For this review, take the finished solid that the model builds, in its own axes (mm). A direction names the side the tool comes from. Coordinates: 2 decimals unless noted, no trailing zeros. Write each loop counter-clockwise with the first axis right and the second up, starting at its lowest first coordinate (ties: lowest second). Pieces come first, ordered by that corner, then holes. Notation, with made-up numbers: (56.5, -31.75) -> (76.5, -31.75) arc R27 ccw to (76.5, -0.75) -> close; hole circle Ø1 at (74.5, -33.75). An arc over 180 degrees is marked (long way). Put each result on its own line as item: value. Start each with the question number.
Item 1: Insertion check: P1, Ø4, axis at x = 7.5, z = -8.5, coming from the +Y side; P2, Ø5, axis at x = 3.5, y = -11.5, coming from the -Z side; P3, Ø6, axis at x = 7, z = -3.5, coming from the -Y side. Each pin has a flat end and moves straight along its axis. Give the tip position at first contact, or say it passes through.
Item 2: For faces 4 (the flat face through (7, -8, -12)), 5 (the cylindrical face through (7.54, 0.07, -10.5)), 6 (the flat face through (0, 0, 8)), 7 (the flat face through (8, 8, -12)), 8 (the flat face through (5, -2, -12)), list the 3-axis set-ups (+Z, -Z, +X, -X, +Y, -Y) from which the entire face can be reached by the end or side of a thin tool; tool diameter is ignored.
Item 3: To check wall thickness, follow L1, parallel to Y at x = 0, z = 5.5; L2, parallel to X at y = -5, z = -18; L3, parallel to Z at x = 2.25, y = -11. State the ranges of each line that lie inside material, in increasing order.
Item 4: Consider section D-D on z = -6.5. Give the boundary of the cut face in (x, y), and give its area (3 significant figures).
Item 5: Consider section B-B on x = 0. Give the boundary of the cut face in (y, z), and give its area (3 significant figures).
Item 6: Consider section C-C on y = 0. Give the boundary of the cut face in (x, z).
Item 7: Consider section A-A on z = -12. Give the boundary of the cut face in (x, y), and give its area (3 significant figures).
Item 8: The part is to be moulded in two halves that separate along Y. For faces 1 (the flat face through (0, 30, 4)), 2 (the cylindrical face through (-7.46, 0.07, -10.5)), 3 (the flat face through (7, 0, -25)), say which applies: +Y half, -Y half, draft (parallel to the pull), parting line (faces both ways), or undercut.
```python
from build123d import *

# Parameters (mm, degrees)
SKETCH_1_W          = 20
SKETCH_1_H          = 60
SKETCH_1_R          = 3
EXTRUDE_1_DEPTH     = 8
EXTRUDE_3_DEPTH     = 25
SKETCH_4_R          = 1.5
CUT_EXTRUDE_1_DEPTH = 25


with BuildPart() as part:
    # 草图1 → 凸台-拉伸1 (new body)
    with BuildSketch(Plane.XY):
        Rectangle(SKETCH_1_W, SKETCH_1_H)
        with Locations((0, 15)):
            Circle(SKETCH_1_R, mode=Mode.SUBTRACT)
        with Locations((0, -15)):
            Circle(SKETCH_1_R, mode=Mode.SUBTRACT)
    extrude(amount=EXTRUDE_1_DEPTH)

    # 草图3 → 凸台-拉伸3 (add)
    with BuildSketch(Plane(origin=(0, 0, 0), x_dir=(-1, 0, 0), z_dir=(0, 0, -1))):
        Polygon((-5, -6), (-5, -8), (-10, -8), (-10, 8), (-5, 8), (-5, 6), align=None)
        Polygon((10, -8), (10, 8), (5, 8), (5, 6), (5, -6), (5, -8), align=None)
    extrude(amount=EXTRUDE_3_DEPTH)

    # 草图4 → 切除-拉伸1 (cut)
    with BuildSketch(Plane(origin=(10, 0, 0), x_dir=(0, 0, -1), z_dir=(1, 0, 0))):
        with Locations((12, 0)):
            Circle(SKETCH_4_R)
    extrude(amount=-CUT_EXTRUDE_1_DEPTH, mode=Mode.SUBTRACT)


solid = part.part
```
Return value:
1. P1: y = 8
1. P2: z = 0
1. P3: y = -8
2. face 4: -Z, +X, -X, -Y
2. face 5: +X, -X
2. face 6: +Z, +X, -X, +Y, -Y
2. face 7: -Z, +X, -X, +Y
2. face 8: -Z, +Y, -Y
3. L1: -30 to -18, -12 to 12, 18 to 30
3. L2: -10 to -5, 5 to 10
3. L3: 0 to 8
4. outline: (-10, -8) -> (-5, -8) -> (-5, 8) -> (-10, 8) -> close; (5, -8) -> (10, -8) -> (10, 8) -> (5, 8) -> close
4. area: 160 mm^2
5. outline: (-30, 0) -> (-18, 0) -> (-18, 8) -> (-30, 8) -> close; (-12, 0) -> (12, 0) -> (12, 8) -> (-12, 8) -> close; (18, 0) -> (30, 0) -> (30, 8) -> (18, 8) -> close
5. area: 384 mm^2
6. outline: (-10, -25) -> (-5, -25) -> (-5, -13.5) -> (-10, -13.5) -> close; (-10, -10.5) -> (-5, -10.5) -> (-5, 0) -> (5, 0) -> (5, -10.5) -> (10, -10.5) -> (10, 8) -> (-10, 8) -> close; (5, -25) -> (10, -25) -> (10, -13.5) -> (5, -13.5) -> close
7. outline: (-10, -8) -> (-5, -8) -> (-5, -1.5) -> (-10, -1.5) -> close; (-10, 1.5) -> (-5, 1.5) -> (-5, 8) -> (-10, 8) -> close; (5, -8) -> (10, -8) -> (10, -1.5) -> (5, -1.5) -> close; (5, 1.5) -> (10, 1.5) -> (10, 8) -> (5, 8) -> close
7. area: 130 mm^2
8. face 1: +Y half
8. face 2: undercut
8. face 3: draft
